Input: part model. Units: mm. Frame: model coordinates. A direction names the side the tool comes from. Round coordinates to 2 decimals unless told otherwise and drop trailing zeros. Loops run counter-clockwise (first coordinate to the right, second up) from the corner with the lowest first, then second, coordinate; pieces in that order, holes last. Notation, with made-up numbers: M 3,-34.75 L 9,-34.75 A35 ccw 9,4.25 Z; hole C -23.5,-25.5 d8. An arc over 180 degrees is marked long. Use one line per item in the form item = value. Start each with the question number.
Q1. Section query C-C, the plane x = 16.25. Output: boundary loops of the cut face in (y, z).
Q2. Access query for faces 5 (the flat face through (16, 2, 3.75)), 6 (the flat face through (32, 2, -1)). Directions: +Z, -Z, +X, -X, +Y, -Y. A direction counts if a zero-diameter tool reaches every point of the face in a straight line with its end or side. Return the directions, or none.
Q3. Ray query, line 1 along X through (y, z) = (3.2, 0); line 2 along Z through (x, y) = (16.25, 2.9); line 3 along X through (y, z) = (2.5, -0.5). Return the intervals inside material, ascending.
Q4. Mould query, pull axis X, two halves, no side actions, for faces 1 (the cylindrical face through (0, 2, 2)), 2 (the cylindrical face through (-3.75, 1.97, 0.08)), 3 (the flat face through (16.5, 4, 2.4)), 4 (the cylindrical face through (36.25, 1.97, -0.08)). Classes: pulls with the +X half, pulls with the -X half, needs draft (parallel to the pull), parting line crosses it, or undercut.
Q5. Section query A-A, the plane z = 0. Output: boundary loops of the cut face in (x, y).
Q6. Section query B-B, the plane y = 1.4. Output: boundary loops of the cut face in (x, z).
Q7. Section query D-D, the plane z = 3. Output: boundary loops of the cut face in (x, y).
```python
from build123d import *

# Parameters (mm, degrees)
SKETCH1_R           = 2
BOSS_EXTRUDE1_DEPTH = 4


with BuildPart() as part:
    # Sketch1 → Boss-Extrude1 (new body)
    with BuildSketch(Plane(origin=(0, 0, 0), x_dir=(1, 0, 0), z_dir=(0, 1, 0))):
        with BuildLine():
            Line((0, 3.75), (32.5, 3.75))
            ThreePointArc((32.5, 3.75), (36.25, 0), (32.5, -3.75))
            Line((32.5, -3.75), (0, -3.75))
            ThreePointArc((0, -3.75), (-3.75, 0), (0, 3.75))
        make_face()
        Circle(SKETCH1_R, mode=Mode.SUBTRACT)
        with Locations((16.25, 0)):
            Circle(SKETCH1_R, mode=Mode.SUBTRACT)
        with BuildLine():
            Line((31.063859338, 1), (33.936140662, 1))
            ThreePointArc((33.936140662, 1), (32.5, -1.75), (31.063859338, 1))
        make_face(mode=Mode.SUBTRACT)
    extrude(amount=BOSS_EXTRUDE1_DEPTH)


solid = part.part
```
Results found:
q1.outline = M 0,-3.75 L 4,-3.75 L 4,-2 L 0,-2 Z; M 0,2 L 4,2 L 4,3.75 L 0,3.75 Z
q2.face_5 = +Z, +X, -X, +Y, -Y
q2.face_6 = +Y, -Y
q3.line_1 = -3.75 to -2, 2 to 14.25, 18.25 to 30.75, 34.25 to 36.25
q3.line_2 = -3.75 to -2, 2 to 3.75
q3.line_3 = -3.72 to -1.94, 1.94 to 14.31, 18.19 to 30.82, 34.18 to 36.22
q4.face_1 = undercut
q4.face_2 = pulls with the -X half
q4.face_3 = needs draft
q4.face_4 = pulls with the +X half
q5.outline = M -3.75,0 L -2,0 L -2,4 L -3.75,4 Z; M 2,0 L 14.25,0 L 14.25,4 L 2,4 Z; M 18.25,0 L 30.75,0 L 30.75,4 L 18.25,4 Z; M 34.25,0 L 36.25,0 L 36.25,4 L 34.25,4 Z
q6.outline = M 0,-3.75 L 32.5,-3.75 A3.75 ccw 32.5,3.75 L 0,3.75 A3.75 ccw Z; hole C 0,0 d4; hole C 16.25,0 d4; hole M 31.06,-1 L 33.94,-1 A1.75 ccw long Z
q7.outline = M -2.25,0 L 34.75,0 L 34.75,4 L -2.25,4 Z
